For this review, take the finished solid that the model builds, in its own axes (mm). A direction names the side the tool comes from. Give positions to 0.01 mm unless a question says otherwise; leave off trailing zeros. Write each loop counter-clockwise with the first axis right and the second up, starting at its lowest first coordinate (ties: lowest second). Pieces come first, ordered by that corner, then holes. Notation, with made-up numbers: (60, -11.75) -> (91, -11.75) arc R34 cw to (91, 27.25) -> close; hole circle Ø5 at (82.25, -31). An arc over 180 degrees is marked (long way). Write item = value, one per line.
```python
from build123d import *

# Parameters (mm, degrees)
SKETCH1_W                   = 7.62
SKETCH1_H                   = 11.43
BOSS_EXTRUDE1_DEPTH         = 7.62
SKETCH2_R                   = 3.499999985
BOSS_EXTRUDE2_DEPTH         = 14.8336
TAP_DRILL_FOR_M4X0_7_TAP1_D = 3.3
FILLET1_R                   = 2.032


with BuildPart() as part:
    # Sketch1 → Boss-Extrude1 (new body)
    with BuildSketch(Plane(origin=(0, 0, 0), x_dir=(0, 1, 0), z_dir=(0, 0, 1))):
        with Locations((-3.81, 5.715)):
            Rectangle(SKETCH1_W, SKETCH1_H)
    extrude(amount=BOSS_EXTRUDE1_DEPTH)

    # Sketch2 → Boss-Extrude2 (add)
    with BuildSketch(Plane.XY.offset(7.62)):
        with Locations((-6.35, -3.81)):
            Circle(SKETCH2_R)
    extrude(amount=BOSS_EXTRUDE2_DEPTH)

    # Tap Drill for M4x0.7 Tap1 (through all)
    with Locations(Plane(origin=(0, 0, 0), x_dir=(0, 0, -1), z_dir=(1, 0, 0))):
        with Locations((-3.81, -3.81)):
            Hole(TAP_DRILL_FOR_M4X0_7_TAP1_D / 2)

    # Fillet1
    fillet1_edges = [part.edges().sort_by_distance(p)[0] for p in [
        (-5.715, -7.62, 0),
        (-5.715, 0, 0),
    ]]
    fillet(fillet1_edges, radius=FILLET1_R)


solid = part.part
```
(1) Take a section at C-C (x = -6.35). Write out the cut boundary in (y, z), plus the area to 3 significant figures.
Answers below:
outline = (-7.62, 2.03) arc R2.03 ccw to (-5.59, 0) -> (-2.03, 0) arc R2.03 ccw to (0, 2.03) -> (0, 7.62) -> (-0.31, 7.62) -> (-0.31, 22.45) -> (-7.31, 22.45) -> (-7.31, 7.62) -> (-7.62, 7.62) -> close; hole circle Ø3.3 at (-3.81, 3.81)
area = 152 mm^2
(2) Take a section at A-A (z = 3.81). Write out the cut boundary in (x, y), plus the area to 3 significant figures.
Answers below:
outline = (-11.43, -7.62) -> (0, -7.62) -> (0, -5.46) -> (-11.43, -5.46) -> close; (-11.43, -2.16) -> (0, -2.16) -> (0, 0) -> (-11.43, 0) -> close
area = 49.4 mm^2
(3) Tool access review of faces 1 (the face through (0, -6, 4)), 2 (the face through (-9.847, -3.656, 14.933)): name each direction out of +Z, -Z, +X, -X, +Y, -Y from which nothing blocks a thin tool from reaching the whole face with its end or side.
Answers below:
face_1 = +Z, -Z, +X, +Y, -Y
face_2 = +Z
(4) Take a section at D-D (z = 8.25). Write out the cut boundary in (x, y), plus the area to 3 significant figures.
Answers below:
outline = circle Ø7 at (-6.35, -3.81)
area = 38.5 mm^2
(5) Take a section at B-B (y = -3.81). Write out the cut boundary in (x, z).
Answers below:
outline = (-11.43, 0) -> (0, 0) -> (0, 2.16) -> (-11.43, 2.16) -> close; (-11.43, 5.46) -> (0, 5.46) -> (0, 7.62) -> (-2.85, 7.62) -> (-2.85, 22.45) -> (-9.85, 22.45) -> (-9.85, 7.62) -> (-11.43, 7.62) -> close
(6) For pin 1 (2.5 mm diameter, centred on y = -3.81, z = 3.81, fed in from +X); pin 2 (2 mm diameter, centred on x = -10, z = 11, fed in from +Y), all flat-tipped, find the tip position at first contact; note any pin that passes through.
Answers below:
pin_1 = through
pin_2 = -1.52
(7) To check wall thickness, follow probe 1 along Y at (x, z) = (-3.75, 3.81); probe 2 along Y at (x, z) = (-1.25, 4.75); probe 3 along Z at (x, y) = (-2, -5). State the ranges of each line that lie inside material, in increasing order.
Answers below:
probe_1 = -7.62 to -5.46, -2.16 to 0
probe_2 = -7.62 to -5.17, -2.45 to 0
probe_3 = 0 to 2.67, 4.95 to 7.62
